from build123d import *

# Parameters (mm, degrees)
F1_DEPTH = 12.7


with BuildPart() as f1:
    # F0 (on Top) → F1 (new body)
    with BuildSketch(Plane.XY):
        Polygon((-31.120982, 6.245733), (-44.473931, 6.245733), (-44.473931, 0), (35.643756, 0), (35.643756, 6.245733), (30.905612, 6.245733), (0, 6.245733), align=None)
        Polygon((0, 32.30552), (-31.120982, 6.245733), (0, 6.245733), align=None)
        Polygon((30.905612, 8.399435), (30.905612, 6.245733), (35.643756, 6.245733), align=None)
    extrude(amount=F1_DEPTH)


solid = f1.part
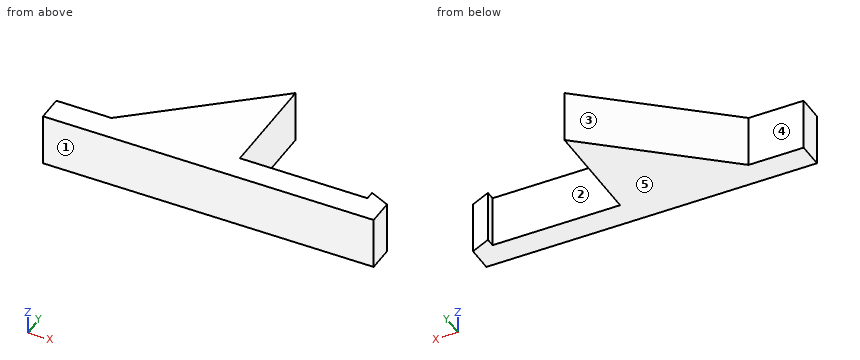
For this review, take the finished solid that the model builds, in its own axes (mm). Face numbers are marked on the shaded views. A direction names the side the tool comes from. Round coordinates to 2 decimals unless told otherwise and drop trailing zeros. Order: outer loops, then holes, each group sorted by start corner. A loop starts at its lowest first (then second) coordinate and runs counter-clockwise, first axis right, second up. Notation, with made-up numbers: (10, 23.5) -> (14, 23.5) arc R25 cw to (14, 58.5) -> close; hole circle Ø2 at (-37.75, 25.25). An arc over 180 degrees is marked (long way). Write item = value, one per line. Start each with the question number.
1) Insertion check: pin 1 (1 mm diameter, centred on y = 12, z = 1.5, fed in from -X); pin 2 (6.5 mm diameter, centred on x = -38, z = 9, fed in from +Y); pin 3 (6 mm diameter, centred on x = -30, z = 8, fed in from -Y); pin 4 (2 mm diameter, centred on y = 28, z = 5.5, fed in from +X). Each pin has a flat end and moves straight along its axis. Give the tip position at first contact, or say it passes through.
2) Take a section at A-A on z = 6.75. State the section outline as (x, y) points, plus the area to 3 significant figures.
3) To check wall thickness, follow line 1 (Y direction, x = 26, z = 10.75); line 2 (Y direction, x = -19.5, z = 3.75); line 3 (X direction, y = 19, z = 10.75). State the ranges of each line that lie inside material, in increasing order. Write a range as from..to.
4) Take a section at B-B on x = 20.5. State the section outline as (y, z) points, plus the area to 3 significant figures.
5) The part is to be moulded in two halves that separate along X. For the marked faces 1, 2 and 3, say which applies: +X half, -X half, draft (parallel to the pull), parting line (faces both ways), or undercut.
6) Tool access review of the marked faces 4 and 5: name each direction out of +Z, -Z, +X, -X, +Y, -Y from which nothing blocks a thin tool from reaching the whole face with its end or side.
7) Take a section at C-C on y = 22. State the section outline as (x, z) points.
Verdict:
q1.pin_1 = -24.85
q1.pin_2 = 6.25
q1.pin_3 = 0
q1.pin_4 = 0
q2.outline = (-44.47, 0) -> (35.64, 0) -> (35.64, 6.25) -> (30.91, 8.4) -> (30.91, 6.25) -> (0, 6.25) -> (0, 32.31) -> (-31.12, 6.25) -> (-44.47, 6.25) -> close
q2.area = 911 mm2
q3.line_1 = 0..6.25
q3.line_2 = 0..15.98
q3.line_3 = -15.89..0
q4.outline = (0, 0) -> (6.25, 0) -> (6.25, 12.7) -> (0, 12.7) -> close
q4.area = 79.3 mm2
q5.face_1 = draft
q5.face_2 = undercut
q5.face_3 = -X half
q6.face_4 = +Z, -Z, -X, +Y
q6.face_5 = -Z, +X, -X, +Y, -Y
q7.outline = (-12.31, 0) -> (0, 0) -> (0, 12.7) -> (-12.31, 12.7) -> close
